from build123d import *

# Parameters (mm, degrees)
SKETCH_1_W          = 12.6
SKETCH_1_H          = 13.45
EXTRUDE_1_DEPTH     = 5.8
FILLET_1_R          = 1.26
SKETCH_2_W          = 5.5
SKETCH_2_H          = 2.5
CUT_EXTRUDE_1_DEPTH = 0.15
SKETCH_4_W          = 5.25
SKETCH_4_H          = 0.075
CUT_EXTRUDE_2_DEPTH = 3.2


with BuildPart() as part:
    # 草图1 → 凸台-拉伸1 (new body)
    with BuildSketch(Plane(origin=(0, 0, 0), x_dir=(1, 0, 0), z_dir=(0, 1, 0))):
        Rectangle(SKETCH_1_W, SKETCH_1_H)
    extrude(amount=EXTRUDE_1_DEPTH)

    # 圆角1
    fillet_1_edges = [part.edges().sort_by_distance(p)[0] for p in [
        (6.3, 2.9, 6.725),
        (-6.3, 2.9, 6.725),
        (-6.3, 2.9, -6.725),
        (6.3, 2.9, -6.725),
    ]]
    fillet(fillet_1_edges, radius=FILLET_1_R)

    # 草图2 → 切除-拉伸1 (cut)
    with BuildSketch(Plane.XZ):
        with Locations((0, 5.475)):
            Rectangle(SKETCH_2_W, SKETCH_2_H)
        with Locations((0, -5.475)):
            Rectangle(SKETCH_2_W, SKETCH_2_H)
    extrude(amount=-CUT_EXTRUDE_1_DEPTH, mode=Mode.SUBTRACT)

    # 切除-扫描1: sweep along a curve in space
    with BuildLine() as sweep_1_path:
        ThreePointArc((-6.3, 5.8, 5.465), (-5.930954544, 5.8, 6.355954544), (-5.04, 5.8, 6.725))
        Line((-5.04, 5.8, 6.725), (5.04, 5.8, 6.725))
        ThreePointArc((5.04, 5.8, 6.725), (5.930954544, 5.8, 6.355954544), (6.3, 5.8, 5.465))
        Line((6.3, 5.8, 5.465), (6.3, 5.8, -5.465))
        ThreePointArc((6.3, 5.8, -5.465), (5.930954544, 5.8, -6.355954544), (5.04, 5.8, -6.725))
        Line((5.04, 5.8, -6.725), (-5.04, 5.8, -6.725))
        ThreePointArc((-5.04, 5.8, -6.725), (-5.930954544, 5.8, -6.355954544), (-6.3, 5.8, -5.465))
        Line((-6.3, 5.8, -5.465), (-6.3, 5.8, 5.465))
    # 草图3 → 切除-扫描1 (sweep, cut)
    with BuildSketch(Plane(origin=(-5.04, 0, 0), x_dir=(0, 0, -1), z_dir=(1, 0, 0))):
        with BuildLine():
            Line((-6.095, 5.8), (-6.725, 5.8))
            Line((-6.725, 5.8), (-6.725, 5.485))
            add(Edge.make_bspline(
                [(-6.095, 5.8), (-6.115272631, 5.8), (-6.369249056, 5.757113449), (-6.508171408, 5.59551094), (-6.709225012, 5.485), (-6.725, 5.485)],
                knots=[0, 0, 0, 0, 0.46408315, 0.583014262, 1, 1, 1, 1], degree=3))
        make_face()
    sweep_1 = sweep(path=sweep_1_path.line, mode=Mode.SUBTRACT)

    # 镜向1: 切除-扫描1 across plane
    add(sweep_1.mirror(Plane.ZX.offset(2.9)), mode=Mode.SUBTRACT)

    # 草图4 → 切除-拉伸2 (cut)
    with BuildSketch(Plane(origin=(0, 0.15, 0), x_dir=(1, 0, 0), z_dir=(0, 1, 0))):
        with Locations((0, -6.6875)):
            Rectangle(SKETCH_4_W, SKETCH_4_H)
    cut_extrude_2 = extrude(amount=CUT_EXTRUDE_2_DEPTH, mode=Mode.SUBTRACT)

    # 镜向2: 切除-拉伸2 across plane
    add(cut_extrude_2.mirror(Plane.XY), mode=Mode.SUBTRACT)


solid = part.part
Could you check a few things on this model? Use its own coordinates, in mm. A direction names the side the tool comes from. Give positions to 0.01 mm unless a question says otherwise; leave off trailing zeros.
1. We'd pull the mould along X, two halves only. Please class faces 1 (the flat face through (0, 2, 6.65)), 2 (the flat face through (0, 5.8, 0)), 3 (the flat face through (0, 0.15, -5)), 4 (the flat face through (-6.3, 3, 0)): pulls with the +X half, pulls with the -X half, needs draft (parallel to the pull), parting line crosses it, or undercut.
2. For faces 5 (the flat face through (0, 4, -6.725)), 6 (the flat face through (0, 2, -6.65)), 7 (the flat face through (0, 0.15, 5)), which set-ups out of +Z, -Z, +X, -X, +Y, -Y let a thin tool reach every point of the face, with its end or its side?
3. Will these pins go through, and if not, where does the flat tip stop? P1, Ø1.8, axis at x = -1, z = 5.5, coming from the -Y side; P2, Ø5, axis at x = -4.5, z = 0.5, coming from the -Y side; P3, Ø1.5, axis at x = 1, y = 1, coming from the +Z side; P4, Ø1.5, axis at x = -1.5, y = 1, coming from the -Z side.
4. I need wall thicknesses on L1, parallel to Z at x = -2, y = 0.85; L2, parallel to Y at x = 1.25, z = 5.75; L3, parallel to X at y = 1.25, z = 6.25. Which ranges of each line are inside material? Lowest first, please.
Solved:
1. face 1: undercut
1. face 2: needs draft
1. face 3: undercut
1. face 4: pulls with the -X half
2. face 5: -Z, +X, -X, +Y, -Y
2. face 6: -Z, -Y
2. face 7: +Z, -Y
3. P1: stops at y = 0.15
3. P2: stops at y = 0
3. P3: stops at z = 6.65
3. P4: stops at z = -6.65
4. L1: z = -6.65 to 6.65
4. L2: y = 0.15 to 5.8
4. L3: x = -6.03 to 6.03
